Geometry: final body of the model. Coordinates: model frame, mm. Face numbers are marked on the shaded views. A direction names the side the tool comes from. Coordinates: 2 decimals unless noted, no trailing zeros. Loops run counter-clockwise (first coordinate to the right, second up) from the corner with the lowest first, then second, coordinate; pieces in that order, holes last. Notation, with made-up numbers: (-37, 19) - (16, 19) arc R7 ccw to (16, 26) - close; hole circle Ø11 at (38, 29.5). An arc over 180 degrees is marked (long way). Write each question's results on one line, items separated by ' | '. Start each with the question number.
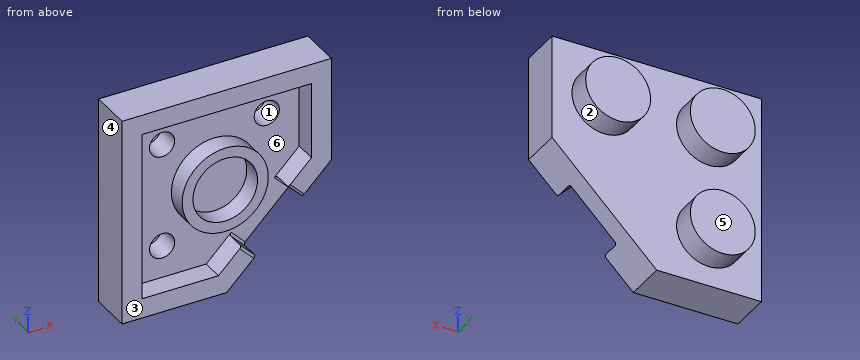
from build123d import *

# Parameters (mm, degrees)
SKETCH1_W               = 15.8
SKETCH1_H               = 15.8
BOSS_EXTRUDE1_DEPTH     = 3.15
SKETCH2_R               = 2.45
BOSS_EXTRUDE2_DEPTH     = 1.85
CUT_EXTRUDE1_DEPTH      = 12.607863714
CUT_EXTRUDE1_DEPTH_BACK = 12.607863714
SHELL1_T                = -1.5
SKETCH4_W               = 5
SKETCH4_H               = 1.65
CUT_EXTRUDE2_DEPTH      = 1.5
FILLET1_R               = 0.2
SKETCH5_R               = 3.25
SKETCH5_R_2             = 2.44
BOSS_EXTRUDE3_DEPTH     = 1.45


with BuildPart() as part:
    # Sketch1 → Boss-Extrude1 (new body)
    with BuildSketch(Plane(origin=(0, 0, 0), x_dir=(1, 0, 0), z_dir=(0, 1, 0))):
        Rectangle(SKETCH1_W, SKETCH1_H)
    extrude(amount=-BOSS_EXTRUDE1_DEPTH)

    # Sketch2 → Boss-Extrude2 (add)
    with BuildSketch(Plane(origin=(0, 0, 0), x_dir=(1, 0, 0), z_dir=(0, 1, 0))):
        with Locations(Location((-3.95, 3.95, 0), (0, 0, 270))):
            Circle(SKETCH2_R)
        with Locations(Location((-3.95, -3.95, 0), (0, 0, 270))):
            Circle(SKETCH2_R)
        with Locations(Location((3.95, -3.95, 0), (0, 0, 270))):
            Circle(SKETCH2_R)
    extrude(amount=BOSS_EXTRUDE2_DEPTH)

    # Sketch3 → Cut-Extrude1 (cut, two sides: drawn at the far end of the back side and taken through both)
    with BuildSketch(Plane(origin=(0, 0, 0), x_dir=(1, 0, 0), z_dir=(0, 1, 0)).offset(-CUT_EXTRUDE1_DEPTH_BACK)):
        Polygon((0, 7.9), (7.9, 0), (7.9, 7.9), align=None)
    extrude(amount=CUT_EXTRUDE1_DEPTH + CUT_EXTRUDE1_DEPTH_BACK, mode=Mode.SUBTRACT)

    # Shell1
    shell1_openings = [part.faces().sort_by_distance(p)[0] for p in [
        (-0.752380952, -3.15, 0.752380952),
    ]]
    offset(amount=SHELL1_T, openings=shell1_openings, kind=Kind.INTERSECTION)

    # Sketch4 → Cut-Extrude2 (cut)
    with BuildSketch(Plane(origin=(3.95, 0, -3.95), x_dir=(-0.7071067811865475, 0, -0.7071067811865477), z_dir=(0.7071067811865477, 0, -0.7071067811865475))):
        with Locations((0, -2.325)):
            Rectangle(SKETCH4_W, SKETCH4_H)
    extrude(amount=-CUT_EXTRUDE2_DEPTH, mode=Mode.SUBTRACT)

    # Fillet1
    fillet1_edges = [part.edges().sort_by_distance(p)[0] for p in [
        (5.187436867, -3.15, -1.651902961),
        (5.187436867, -1.5, -1.651902961),
        (1.651902961, -1.5, -5.187436867),
        (1.651902961, -3.15, -5.187436867),
    ]]
    fillet(fillet1_edges, radius=FILLET1_R)

    # Sketch5 → Boss-Extrude3 (add)
    with BuildSketch(Plane.XZ.offset(1.5)):
        with Locations(Location((0, 0, 0), (0, 0, 90))):
            Circle(SKETCH5_R)
        with Locations(Location((0, 0, 0), (0, 0, 90))):
            Circle(SKETCH5_R_2, mode=Mode.SUBTRACT)
    extrude(amount=BOSS_EXTRUDE3_DEPTH)


solid = part.part
1) Section query A-A on y = -1.1. Output: boundary loops of the cut face in (x, z).
2) Section query D-D on y = 1.1. Output: boundary loops of the cut face in (x, z).
3) Material intervals for line 1 (Z direction, x = -3.95, y = -0.5); line 2 (Z direction, x = 1.75, y = -2.35), sorted ascending. Write a range as [from, to].
4) Pull-direction query (X, two-part tool) for the marked faces 4, 5 and 6; classes: released by +X, released by -X, zero draft, split by the parting line, or undercut.
5) Pin query (flat end, axial travel): pin 1 Ø6.5 at (x, z) = (-2.5, -1) entering from -Y; pin 2 Ø1.5 at (x, z) = (-4.5, 4) entering from -Y; pin 3 Ø0.6 at (x, z) = (-4.5, -4) entering from -Y. Return the tip coordinate at first contact, or that it passes through.
6) Section query C-C on x = 3.95. Output: boundary loops of the cut face in (y, z).
7) Section query B-B on z = 3.95. Output: boundary loops of the cut face in (x, y), and give its area (4 significant figures).
8) Access query for the marked faces 1, 2 and 3. Directions: +Z, -Z, +X, -X, +Y, -Y. A direction counts if a zero-diameter tool reaches every point of the face in a straight line with its end or side. Return the directions, or none.
Returned:
1) outline: (-7.9, -7.9) - (0, -7.9) - (7.9, 0) - (7.9, 7.9) - (-7.9, 7.9) - close; hole circle Ø1.9 at (-3.95, -3.95); hole circle Ø1.9 at (-3.95, 3.95); hole circle Ø1.9 at (3.95, 3.95)
2) outline: circle Ø4.9 at (-3.95, -3.95); circle Ø4.9 at (-3.95, 3.95); circle Ø4.9 at (3.95, 3.95)
3) line 1: z = [-7.9, -4.9], [-3, 3], [4.9, 7.9] | line 2: z = [-6.15, -5.29], [-2.74, -1.7], [1.7, 2.74], [6.4, 7.9]
4) face 4: released by -X | face 5: zero draft | face 6: undercut
5) pin 1: stops at y = -2.95 | pin 2: stops at y = -1.5 | pin 3: stops at y = 0.35
6) outline: (-3.15, 6.4) - (-1.5, 6.4) - (-1.5, 4.9) - (0.35, 4.9) - (0.35, 3) - (-1.5, 3) - (-1.5, -3.95) - (0, -3.95) - (0, 1.5) - (1.85, 1.5) - (1.85, 6.4) - (0, 6.4) - (0, 7.9) - (-3.15, 7.9) - close
7) outline: (-7.9, -3.15) - (-6.4, -3.15) - (-6.4, -1.5) - (-4.9, -1.5) - (-4.9, 0.35) - (-3, 0.35) - (-3, -1.5) - (3, -1.5) - (3, 0.35) - (4.9, 0.35) - (4.9, -1.5) - (6.4, -1.5) - (6.4, -3.15) - (7.9, -3.15) - (7.9, 0) - (6.4, 0) - (6.4, 1.85) - (1.5, 1.85) - (1.5, 0) - (-1.5, 0) - (-1.5, 1.85) - (-6.4, 1.85) - (-6.4, 0) - (-7.9, 0) - close | area: 39.75 mm²
8) face 1: -Y | face 2: +Y | face 3: +Z, -Z, +X, -X, -Y
